Work out the finished part from the listing and answer in its coordinate system (mm). A direction names the side the tool comes from. Round coordinates to 2 decimals unless told otherwise and drop trailing zeros. Loops run counter-clockwise (first coordinate to the right, second up) from the corner with the lowest first, then second, coordinate; pieces in that order, holes last.
```python
from build123d import *

# Parameters (mm, degrees)
SALIENTE_EXTRUIR1_DEPTH = 60
CROQUIS3_R              = 2.5
CORTAR_EXTRUIR1_DEPTH   = 60
CROQUIS4_R              = 2
CROQUIS4_W              = 20
CROQUIS4_H              = 40
CORTAR_EXTRUIR2_DEPTH   = 60


with BuildPart() as part:
    # Croquis2 → Saliente-Extruir1 (new body)
    with BuildSketch(Plane.XY):
        Polygon((-27.386914876, 0), (12.613085124, 0), (12.613085124, 2), (-25.386914876, 2), (-25.386914876, 12), (-27.386914876, 12), align=None)
    extrude(amount=SALIENTE_EXTRUIR1_DEPTH)

    # Croquis3 → Cortar-Extruir1 (cut)
    with BuildSketch(Plane.ZY.offset(27.386914876)):
        with Locations((10, 6)):
            Circle(CROQUIS3_R)
        with Locations((50, 6)):
            Circle(CROQUIS3_R)
    extrude(amount=-CORTAR_EXTRUIR1_DEPTH, mode=Mode.SUBTRACT)

    # Croquis4 → Cortar-Extruir2 (cut)
    with BuildSketch(Plane.XZ):
        with Locations((-7.386914876, 55)):
            Circle(CROQUIS4_R)
        with Locations((2.613085124, 55)):
            Circle(CROQUIS4_R)
        with Locations((-7.386914876, 5)):
            Circle(CROQUIS4_R)
        with Locations((2.613085124, 5)):
            Circle(CROQUIS4_R)
        with Locations((-2.386914876, 30)):
            Rectangle(CROQUIS4_W, CROQUIS4_H)
    extrude(amount=-CORTAR_EXTRUIR2_DEPTH, mode=Mode.SUBTRACT)


solid = part.part
```
1. Find section D-D (z = 42). Write down the section's boundary in (x, y).
Answer key:
outline: (-27.39, 0) - (-12.39, 0) - (-12.39, 2) - (-25.39, 2) - (-25.39, 12) - (-27.39, 12) - close; (7.61, 0) - (12.61, 0) - (12.61, 2) - (7.61, 2) - close
2. Given pin 1 (19 mm diameter, centred on x = -11, z = 18.5, fed in from +Y); pin 2 (10 mm diameter, centred on x = 1, z = 35.5, fed in from -Y); pin 3 (3 mm diameter, centred on y = 5.5, z = 22, fed in from +X), each flat-ended and moving along its own axis, determine where each tip first touches the part or whether it passes through.
Answer key:
pin 1: stops at y = 2
pin 2: passes through
pin 3: stops at x = -25.39
3. Which of the six approach directions +Z, -Z, +X, -X, +Y, -Y give full straight-line access (tool end or side, diameter ignored) to faces 5 (the face through (-3, 1, 10)), 6 (the face through (12.613, 1, 30)), 7 (the face through (-15, 2, 30))?
Answer key:
face 5: +Y, -Y
face 6: +Z, -Z, +X, +Y, -Y
face 7: +Z, -Z, +X, +Y
4. Find section B-B (x = -1). Write down the section's boundary in (y, z), then the cut area to 3 significant figures.
Answer key:
outline: (0, 0) - (2, 0) - (2, 10) - (0, 10) - close; (0, 50) - (2, 50) - (2, 60) - (0, 60) - close
area: 40.0 mm2
5. Find section A-A (z = 5). Write down the section's boundary in (x, y).
Answer key:
outline: (-27.39, 0) - (-9.39, 0) - (-9.39, 2) - (-25.39, 2) - (-25.39, 12) - (-27.39, 12) - close; (-5.39, 0) - (0.61, 0) - (0.61, 2) - (-5.39, 2) - close; (4.61, 0) - (12.61, 0) - (12.61, 2) - (4.61, 2) - close
6. Determine the mould class of faces 1 (the face through (7.613, 1, 30)), 2 (the face through (-26.4, 8.48, 9.67)), 3 (the face through (-26.401, 6.751, 52.385)), 4 (the face through (-17, 0, 30)) for opening direction Y: +Y half, -Y half, draft (parallel to the pull), parting line (faces both ways), or undercut.
Answer key:
face 1: draft
face 2: undercut
face 3: undercut
face 4: -Y half
7. Find section C-C (y = 6). Write down the section's boundary in (x, z), then the cut area to 3 significant figures.
Answer key:
outline: (-27.39, 0) - (-25.39, 0) - (-25.39, 7.5) - (-27.39, 7.5) - close; (-27.39, 12.5) - (-25.39, 12.5) - (-25.39, 47.5) - (-27.39, 47.5) - close; (-27.39, 52.5) - (-25.39, 52.5) - (-25.39, 60) - (-27.39, 60) - close
area: 100 mm2
8. Consider probe 1 along Z at (x, y) = (-5, 1); probe 2 along Y at (x, z) = (-21.5, 21.5); probe 3 along X at (y, z) = (3.25, 23). Determine where each line is inside the solid, lowest interval first.
Answer key:
probe 1: z = 0 to 10, 50 to 60
probe 2: y = 0 to 2
probe 3: x = -27.39 to -25.39
